```python
from build123d import *

# Parameters (mm, degrees)
SKETCH3_R   = 3.175
SKETCH6_W   = 6.3
SKETCH6_H   = 5
SKETCH6_W_2 = 5
SKETCH6_H_2 = 6.3
SKETCH6_W_3 = 38.125


with BuildPart() as part:
    # Sketch3 → Revolve1 (revolve)
    with BuildSketch(Plane.XY):
        with Locations((-41.275, 0)):
            Circle(SKETCH3_R)
    revolve(axis=Axis((0, -2.75, 0), (0, 1, 0)))

    # Sketch6 → Cut-Revolve1 (revolve, cut)
    with BuildSketch(Plane.XY):
        with Locations((-41.275, -5.65)):
            Rectangle(SKETCH6_W, SKETCH6_H)
        with Locations((-46.925, 0)):
            Rectangle(SKETCH6_W_2, SKETCH6_H_2)
        with Locations((-41.275, 5.65)):
            Rectangle(SKETCH6_W, SKETCH6_H)
        with Locations((-19.0625, 0)):
            Rectangle(SKETCH6_W_3, SKETCH6_H_2)
    revolve(axis=Axis((0, -2.75, 0), (0, 1, 0)), mode=Mode.SUBTRACT)


solid = part.part
```
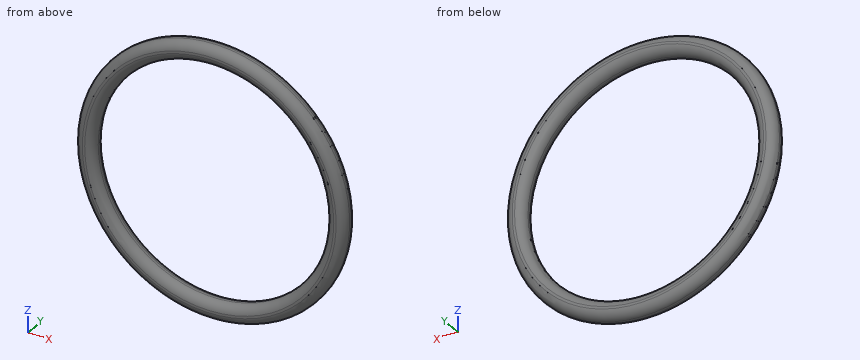
The listing builds one solid part. Answer for the finished solid, in the listing's coordinates (mm). Give positions to 0.01 mm unless a question says otherwise; leave off trailing zeros. Order: outer loops, then holes, each group sorted by start corner. A loop starts at its lowest first (then second) coordinate and runs counter-clockwise, first axis right, second up.
Item 1: The part is cut by section A-A, the plane x = 0. Give the vertices of the cut face in (y, z) (3 decimals), and give its area (3 significant figures).
From the geometry:
outline: (-3.15, -41.673) arc R3.175 ccw to (-0.398, -44.425) - (0.398, -44.425) arc R3.175 ccw to (3.15, -41.673) - (3.15, -40.877) arc R3.175 ccw to (0.398, -38.125) - (-0.398, -38.125) arc R3.175 ccw to (-3.15, -40.877) - close; (-3.15, 40.877) arc R3.175 ccw to (-0.398, 38.125) - (0.398, 38.125) arc R3.175 ccw to (3.15, 40.877) - (3.15, 41.673) arc R3.175 ccw to (0.398, 44.425) - (-0.398, 44.425) arc R3.175 ccw to (-3.15, 41.673) - close
area: 63.2 mm2
Item 2: Given pin 1 Ø1 at (y, z) = (-2.5, -26.5) entering from +X, flat-ended and moving along its own axis, determine where the tip first touches the part or whether it passes through.
From the geometry:
pin 1: stops at x = 34.92
Item 3: The part is cut by section C-C, the plane y = -1.5. Give the vertices of the cut face in (x, z), and give its area (3 significant figures).
From the geometry:
outline: circle Ø88.15 at (0, 0); hole circle Ø76.95 at (0, 0)
area: 1,450 mm2
Item 4: Find the intervals of material crossed by probe 1 along Z at (x, y) = (0, -0.1) (3 decimals); probe 2 along X at (y, z) = (2.5, -23); probe 3 along X at (y, z) = (-2, -1.5), in increasing order.
From the geometry:
probe 1: z = -44.425 to -38.125, 38.125 to 44.425
probe 2: x = -36.61 to -31.89, 31.89 to 36.61
probe 3: x = -43.72 to -38.78, 38.78 to 43.72
Item 5: The part is cut by section B-B, the plane z = 0. Give the vertices of the cut face in (x, y) (3 decimals).
From the geometry:
outline: (-44.425, -0.398) arc R3.175 ccw to (-41.673, -3.15) - (-40.877, -3.15) arc R3.175 ccw to (-38.125, -0.398) - (-38.125, 0.398) arc R3.175 ccw to (-40.877, 3.15) - (-41.673, 3.15) arc R3.175 ccw to (-44.425, 0.398) - close; (38.125, -0.398) arc R3.175 ccw to (40.877, -3.15) - (41.673, -3.15) arc R3.175 ccw to (44.425, -0.398) - (44.425, 0.398) arc R3.175 ccw to (41.673, 3.15) - (40.877, 3.15) arc R3.175 ccw to (38.125, 0.398) - close
